Can you work these out from the model? Positions are in its coordinate system, mm. Give positions to 0.01 mm unless a question says otherwise; leave off trailing zeros. Order: outer loops, then holes, each group sorted by start corner. A loop starts at its lowest first (then second) coordinate and runs counter-clockwise, first axis right, second up. Notation, with made-up numbers: M 86,-9 L 129,-9 A18 cw 129,10 Z; hole C 83.5,-39.5 d4. An arc over 180 degrees is marked long. Answer as a JSON object with one key per item and string values.
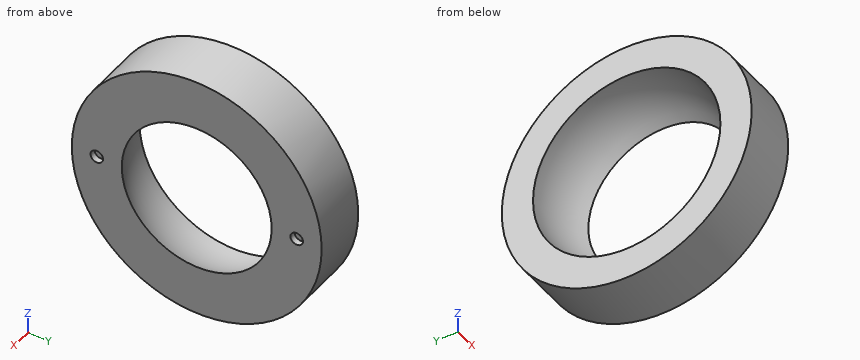
Autodesk Inventor part; units mm, degrees
ref_plane "Work Plane1" through (0, 0, 0) normal (0, 0, 1) x (1, 0, 0)
ref_plane "YZ Plane" through (0, 0, 0) normal (1, 0, 0) x (0, 1, 0)
ref_plane "XZ Plane" through (0, 0, 0) normal (0, 1, 0) x (-1, 0, 0)
ref_plane "Work Plane1" through (0, 0, 0) normal (0, 0, 1) x (1, 0, 0)
sketch "Sketch1" plane through (0, 0, 0) normal (0, 0, 1) x (1, 0, 0)
  line L0 (-8.678, -58.5397) -> (-8.678, 43.8978) construction
  line L1 (1.322, -54.9064) -> (1.322, 43.8978) construction
  circle A0 centre (-8.678, 43.8978) radius 15 construction
  line L2 (-8.678, 23.8978) -> (1.322, 23.8978) construction
  line L3 (0.322, 23.8978) -> (0.322, 31.8978)
  line L4 (-8.678, 28.8978) -> (-8.678, 23.8978)
  line L5 (-8.678, 23.8978) -> (0.322, 23.8978)
  arc A1 (-8.678, 28.8978) -> (0.322, 31.8978) centre (-8.678, 43.8978) ccw
  line L6 (-8.678, 43.8978) -> (1.322, 43.8978) construction
  point P0 (0, 0)
  dimension "d0" = 1
revolve "Revolution1" add sketch "Sketch1" angle 360 about axis through (-8.678, 43.8978, 0) along (1, 0, 0)
thread "Thread2"
sketch "Sketch9" plane through (0.322, 43.8978, 0) normal (1, 0, 0) x (0, 0, -1)
  circle A0 centre (0, 0) radius 12 construction
  circle A1 centre (0, 0) radius 20 construction
  circle A2 centre (0, 0) radius 16 construction
  line L0 (0, -56.6773) -> (0, 32.7796) construction
  circle A3 centre (0, -16) radius 1
  circle A4 centre (0, 16) radius 1
  point P0 (0, -43.8978)
  dimension "d49" = 4
  dimension "d50" = 8
  dimension "d51" = 2
  dimension "d52" = 2
extrude "Extrusion2" cut sketch "Sketch9" against normal blind 1
equation "\"d49\" = 0.5 * d50"
equation "\"d52\" = d51"
equation "\"d11\" = 55deg"
equation "\"Sketch2_Pitch\" = 1.5"
equation "\"d32\" = 55deg"
equation "\"Sketch5_Pitch\" = 1.5"
properties part number "MCEN4000:T6" material "STEEL, AISI 1040"
1) I want a section at D-D on z = 0. Write out the boundary of the cut face in (x, y).
Results found:
{"outline": "M -8.68,23.9 L 0.32,23.9 L 0.32,26.9 L -0.68,26.9 L -0.68,28.9 L 0.32,28.9 L 0.32,31.9 A15 cw -8.68,28.9 Z; M -8.68,58.9 A15 cw 0.32,55.9 L 0.32,58.9 L -0.68,58.9 L -0.68,60.9 L 0.32,60.9 L 0.32,63.9 L -8.68,63.9 Z"}
2) I'm going to push flat-ended pins straight in: pin 1 Ø2 at (x, z) = (-2.5, -14) entering from +Y; pin 2 Ø1 at (x, z) = (-4.5, 13) entering from +Y; pin 3 Ø3 at (x, z) = (-5, -5.5) entering from -Y. Where does each tip first touch, or does it pass through?
Results found:
{"pin 1": "stops at y = 59.1", "pin 2": "stops at y = 59.51", "pin 3": "stops at y = 24.3"}
3) I need wall thicknesses on L1, parallel to Y at x = 0.05, z = 0; L2, parallel to Y at x = -0.2, z = 0; L3, parallel to Z at x = -5.75, y = 45.5. Which ranges of each line are inside material? Lowest first, please.
Results found:
{"L1": "y = 23.9 to 26.9, 28.9 to 31.7, 56.1 to 58.9, 60.9 to 63.9", "L2": "y = 23.9 to 26.9, 28.9 to 31.52, 56.27 to 58.9, 60.9 to 63.9", "L3": "z = -19.94 to -14.62, 14.62 to 19.94"}
4) I want a section at B-B on y = 39. Write out the boundary of the cut face in (x, z), and give its area (3 significant figures).
Results found:
{"outline": "M -8.68,-19.39 L 0.32,-19.39 L 0.32,-10.95 A14.18 cw -8.68,-14.18 Z; M -8.68,14.18 A14.18 cw 0.32,10.95 L 0.32,19.39 L -8.68,19.39 Z", "area": "112 mm²"}
5) I want a section at A-A on z = 8.5. Write out the boundary of the cut face in (x, y).
Results found:
{"outline": "M -8.68,25.79 L 0.32,25.79 L 0.32,35.43 A12.36 cw -8.68,31.54 Z; M -8.68,56.26 A12.36 cw 0.32,52.37 L 0.32,62 L -8.68,62 Z"}
6) I want a section at C-C on x = -1.75. Write out the boundary of the cut face in (y, z), and give its area (3 significant figures).
Results found:
{"outline": "C 43.9,0 d40; hole C 43.9,0 d26.61", "area": "701 mm²"}
